Design review of the part built by this model. Coordinates are the model's own, in mm. A direction names the side the tool comes from. Give positions to 0.01 mm unless a question says otherwise; leave off trailing zeros. Order: outer loops, then holes, each group sorted by start corner. A loop starts at its lowest first (then second) coordinate and runs counter-clockwise, first axis right, second up. Notation, with made-up numbers: (73, 25.5) -> (105, 25.5) arc R38 cw to (105, 63.5) -> close; hole circle Ø11 at (22.5, -8.75). An arc over 180 degrees is marked (long way). One line per item, written item: value. Start each with the question number.
1) For pin 1 (0.8 mm diameter, centred on x = 26.5, y = 6, fed in from -Z); pin 2 (4 mm diameter, centred on x = -28, z = 7, fed in from +Y); pin 3 (4 mm diameter, centred on y = -4.5, z = 7.5, fed in from -X); pin 4 (10 mm diameter, centred on x = 14.5, z = 7, fed in from -Y), all flat-tipped, find the tip position at first contact; note any pin that passes through.
2) The part is to be moulded in two halves that separate along X. For faces 4 (the face through (1, 3.218, 10)), 5 (the face through (-24.959, 0, 10)), 6 (the face through (26, 7.018, 18)), 7 (the face through (25.301, -3, 10)), say which applies: released by +X, released by -X, zero draft, split by the parting line, or undercut.
3) Consider section D-D (x = -14). State the section outline as (y, z) points, plus the area to 3 significant figures.
4) Wall thickness on line 1 along X through (y, z) = (-8.5, 2.5); line 2 along X through (y, z) = (0, 19.5); line 3 along Y through (x, z) = (11.5, 10): over which ranges is each line inside the solid? List them lowest first. Write a range as from..to.
5) Consider section A-A (y = 1.5). State the section outline as (x, z) points.
6) Consider section C-C (x = 30.5). State the section outline as (y, z) points.
7) Tool access review of faces 1 (the face through (-22.959, -3, 10)), 2 (the face through (26, 6, 5)), 3 (the face through (34, -8.064, 10)): name each direction out of +Z, -Z, +X, -X, +Y, -Y from which nothing blocks a thin tool from reaching the whole face with its end or side.
8) Consider section B-B (z = 10.3). State the section outline as (x, y) points.
from build123d import *

# Parameters (mm, degrees)
RESSALTO_EXTRUS_O1_DEPTH = 20.6
ESBO_O2_W                = 48.26
ESBO_O2_H                = 13.2
CORTE_EXTRUS_O1_DEPTH    = 25.4
ESBO_O3_W                = 20.6
ESBO_O3_H                = 1.5
RESSALTO_EXTRUS_O2_DEPTH = 2
ESBO_O4_W                = 5
ESBO_O4_H                = 1.5
RESSALTO_EXTRUS_O3_DEPTH = 2
ESBO_O5_R                = 2.5
CORTE_EXTRUS_O2_DEPTH    = 2


with BuildPart() as part:
    # Esboço1 → Ressalto-extrusão1 (new body)
    with BuildSketch(Plane.XY):
        Polygon((35.300916774, -9.982051282), (-32.959083226, -9.982051282), (-32.959083226, -8.064102564), (-24.959083226, -8.064102564), (-24.959083226, 5.517948718), (27.300916774, 5.517948718), (27.300916774, -8.064102564), (35.300916774, -8.064102564), align=None)
    extrude(amount=RESSALTO_EXTRUS_O1_DEPTH)

    # Esboço2 → Corte-extrusão1 (cut)
    with BuildSketch(Plane.XY.offset(20.6)):
        with Locations((1.170916774, -3.382051282)):
            Rectangle(ESBO_O2_W, ESBO_O2_H)
    extrude(amount=-CORTE_EXTRUS_O1_DEPTH, mode=Mode.SUBTRACT)

    # Esboço3 → Ressalto-extrusão2 (add)
    with BuildSketch(Plane.ZY.offset(24.959083226)):
        with Locations((10.3, 6.267948718)):
            Rectangle(ESBO_O3_W, ESBO_O3_H)
    extrude(amount=-RESSALTO_EXTRUS_O2_DEPTH)

    # Esboço4 → Ressalto-extrusão3 (add)
    with BuildSketch(Plane(origin=(27.300916774, 0, 0), x_dir=(0, 0, -1), z_dir=(1, 0, 0))):
        with Locations((-18.1, 6.267948718)):
            Rectangle(ESBO_O4_W, ESBO_O4_H)
        with Locations((-2.5, 6.267948718)):
            Rectangle(ESBO_O4_W, ESBO_O4_H)
    extrude(amount=-RESSALTO_EXTRUS_O3_DEPTH)

    # Esboço5 → Corte-extrusão2 (cut)
    with BuildSketch(Plane(origin=(0, -8.064102564, 0), x_dir=(1, 0, 0), z_dir=(0, 1, 0))):
        with Locations(Location((-28.959083226, -10.3, 0), (0, 0, 180))):
            Circle(ESBO_O5_R)
        with Locations(Location((31.300916774, -10.3, 0), (0, 0, 180))):
            Circle(ESBO_O5_R)
    extrude(amount=-CORTE_EXTRUS_O2_DEPTH, mode=Mode.SUBTRACT)


solid = part.part
Checked values:
1. pin 1: stops at z = 0
1. pin 2: stops at y = -8.06
1. pin 3: stops at x = -24.96
1. pin 4: stops at y = 3.22
2. face 4: undercut
2. face 5: released by -X
2. face 6: zero draft
2. face 7: undercut
3. outline: (3.22, 0) -> (5.52, 0) -> (5.52, 20.6) -> (3.22, 20.6) -> close
3. area: 47.4 mm^2
4. line 1: x = -32.96..-22.96, 25.3..35.3
4. line 2: x = -24.96..-22.96, 25.3..27.3
4. line 3: y = 3.22..5.52
5. outline: (-24.96, 0) -> (-22.96, 0) -> (-22.96, 20.6) -> (-24.96, 20.6) -> close; (25.3, 0) -> (27.3, 0) -> (27.3, 20.6) -> (25.3, 20.6) -> close
6. outline: (-9.98, 0) -> (-8.06, 0) -> (-8.06, 7.93) -> (-9.98, 7.93) -> close; (-9.98, 12.67) -> (-8.06, 12.67) -> (-8.06, 20.6) -> (-9.98, 20.6) -> close
7. face 1: +Z, -Z, -Y
7. face 2: +X, +Y
7. face 3: +Z, -Z, +X, +Y
8. outline: (-32.96, -9.98) -> (-31.46, -9.98) -> (-31.46, -8.06) -> (-32.96, -8.06) -> close; (-26.46, -9.98) -> (-22.96, -9.98) -> (-22.96, 3.22) -> (25.3, 3.22) -> (25.3, -9.98) -> (28.8, -9.98) -> (28.8, -8.06) -> (27.3, -8.06) -> (27.3, 5.52) -> (-22.96, 5.52) -> (-22.96, 7.02) -> (-24.96, 7.02) -> (-24.96, -8.06) -> (-26.46, -8.06) -> close; (33.8, -9.98) -> (35.3, -9.98) -> (35.3, -8.06) -> (33.8, -8.06) -> close
